For this review, take the finished solid that the model builds, in its own axes (mm). Coordinates: 2 decimals unless noted, no trailing zeros. Order: outer loops, then holes, each group sorted by start corner. A loop starts at its lowest first (then second) coordinate and runs counter-clockwise, first axis right, second up. Notation, with made-up numbers: (2, 64.5) -> (37, 64.5) arc R22 ccw to (37, 72.5) -> close; hole circle Ø3 at (62.25, -12.5). An arc over 180 degrees is marked (long way). Write item = value, one per line. Start each with the question number.
1) Insertion check: pin 1 Ø2 at (x, y) = (10.5, -2.5) entering from -Z; pin 2 Ø2 at (x, y) = (41, -1.5) entering from +Z; pin 3 Ø2 at (x, y) = (27, -4) entering from +Z. Each pin has a flat end and moves straight along its axis. Give the tip position at first contact, or say it passes through.
2) Consider section C-C on x = 20.5. Give the boundary of the cut face in (y, z), and give its area (3 significant figures).
3) Consider section B-B on z = 12. Give the boundary of the cut face in (x, y).
4) Wall thickness on probe 1 along X at (y, z) = (-3.7, -4); probe 2 along X at (y, z) = (-3.6, 15); probe 3 along X at (y, z) = (-0.3, -2.5): over which ranges is each line inside the solid? List them lowest first. Write a range as [from, to].
5) Consider section A-A on y = -1.4. State how many separate pieces and enclosed holes the cut face has, and give its area (3 significant figures).
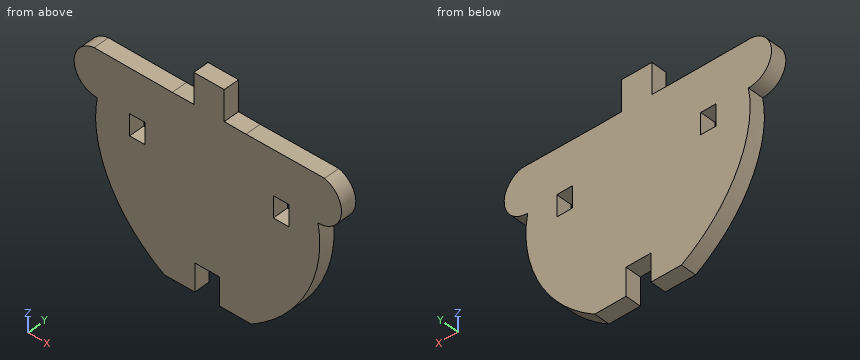
from build123d import *

# Parameters (mm, degrees)
F0_W     = 4.2672
F0_H     = 5.842
F1_DEPTH = 4.3434


with BuildPart() as f1:
    # F0 (on Front) → F1 (new body)
    with BuildSketch(Plane.XZ):
        with BuildLine():
            Line((2.1634316072, 10.8543494716), (-19.3501866255, 10.9726172321))
            ThreePointArc((-19.3501866255, 10.9726172321), (-24.8410026739, 4.2145660489), (-18.4759762851, -1.7273827679))
            add(Edge.make_bspline(
                [(-18.4759762851, -1.7273827679), (-20.8852616932, -14.0894673655), (-14.3136853987, -29.476307077), (0, -38.1591799864)],
                knots=[0, 0, 0, 0, 0.1710209887, 0.1710209887, 0.1710209887, 0.1710209887], degree=3))
            Line((0, -38.1591799864), (8.3743836731, -38.1230656058))
            Line((8.3743836731, -38.1230656058), (8.3743836731, -30.5030656058))
            Line((8.3743836731, -30.5030656058), (12.2675002734, -30.5030656058))
            Line((12.2675002734, -30.5030656058), (15.2323836731, -30.5030656058))
            Line((15.2323836731, -30.5030656058), (15.2323836731, -38.1230656058))
            Line((15.2323836731, -38.1230656058), (23.8656476492, -38.1591799864))
            add(Edge.make_bspline(
                [(42.3416239343, -1.7273827679), (44.7509093424, -14.0894673655), (38.1793330479, -29.476307077), (23.8656476492, -38.1591799864)],
                knots=[0, 0, 0, 0, 0.1710209887, 0.1710209887, 0.1710209887, 0.1710209887], degree=3))
            ThreePointArc((42.3416239343, -1.7273827679), (48.7556622303, 3.8381273274), (44.1498133745, 10.9726172321))
            Line((44.1498133745, 10.9726172321), (22.4834316072, 10.8543494716))
            Line((22.4834316072, 10.8543494716), (16.4287500314, 10.9232757241))
            Line((16.4287500314, 10.9232757241), (16.4984082512, 10.9232757241))
            Line((16.4984082512, 10.9232757241), (16.4984082512, 19.3052757241))
            Line((16.4984082512, 19.3052757241), (8.1164082512, 19.3052757241))
            Line((8.1164082512, 19.3052757241), (8.1164082512, 10.9232757241))
            Line((8.1164082512, 10.9232757241), (8.294825498, 10.9232757241))
            Line((8.294825498, 10.9232757241), (2.1634316072, 10.8543494716))
        make_face()
        with Locations((-7.4751781712, -3.9884169885)):
            Rectangle(F0_W, F0_H, mode=Mode.SUBTRACT)
        Polygon((30.0267527077, -7.0222468014), (30.0640258865, -1.180365708), (34.331139033, -1.2075913342), (34.2938658543, -7.0494724276), align=None, mode=Mode.SUBTRACT)
    extrude(amount=F1_DEPTH)


solid = f1.part
Answer sheet:
q1.pin_1 = -30.5
q1.pin_2 = 10.96
q1.pin_3 = 10.88
q2.outline = (-4.34, -38.15) -> (0, -38.15) -> (0, 10.88) -> (-4.34, 10.88) -> close
q2.area = 213 mm2
q3.outline = (8.12, -4.34) -> (16.5, -4.34) -> (16.5, 0) -> (8.12, 0) -> close
q4.probe_1 = [-18.81, -9.61], [-5.34, 30.05], [34.31, 42.68]
q4.probe_2 = [8.12, 16.5]
q4.probe_3 = [-18.61, -9.61], [-5.34, 30.06], [34.32, 42.48]
q5.separate_pieces = 1
q5.enclosed_holes = 2
q5.area = 2,760 mm2
